Can you work these out from the drawing? Everything is in mm from the part's minimum corner. Coordinates: 2 decimals unless noted, no trailing zeros. Order: outer loops, then holes, each group sorted by start corner. A loop starts at its lowest first (then second) coordinate and runs counter-clockwise, first axis right, second up. Notation, with made-up numbers: (42.5, 34) -> (78.5, 34) arc R19 cw to (78.5, 68) -> close; hole circle Ø4 at (-9.75, 19). An arc over 180 degrees is marked (long way). Return JSON: item names as keys, results as strings. Group by question number.
1) If we section it at D-D, the plane x = 6: Please give me the cut outline in (y, z), then the cut area to 3 significant figures.
2) If I drill on probe 1 along Y at (x, z) = (6, 0.7); probe 2 along Y at (x, z) = (4, 1.15); probe 3 along X at (y, z) = (21.25, 1.8), over which ranges is the centre line in solid material (lowest first)? Write a range as from..to.
3) For pin 1 (4.5 mm diameter, centred on x = 4, y = 20, fed in from +Z); pin 2 (4 mm diameter, centred on x = 15, y = 25, fed in from -Z), each with a flat end and sliding along its axis, tell me the tip position at first contact or that it passes through.
4) If we section it at C-C, the plane y = 25.5: Please give me the cut outline in (x, z), then the cut area to 3 significant figures.
5) If we section it at A-A, the plane x = 36: Please give me the cut outline in (y, z), then the cut area to 3 significant figures.
6) Thinking about a two-plate mould opening in Y: for the marked faces 1, 2 and 3, which applies, +Y half, -Y half, draft (parallel to the pull), parting line (faces both ways), or undercut?
7) If we section it at B-B, the plane z = 1.1: Please give me the cut outline in (x, y).
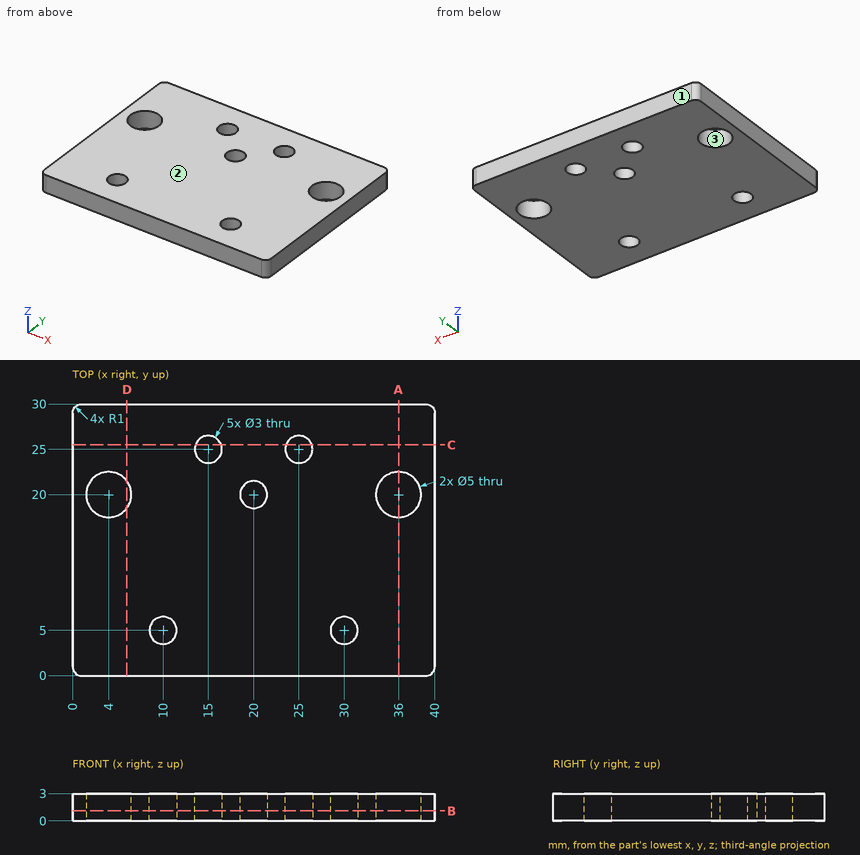
Result sheet:
{
 "1": {"outline": "(0, 0) -> (18.5, 0) -> (18.5, 3) -> (0, 3) -> close; (21.5, 0) -> (30, 0) -> (30, 3) -> (21.5, 3) -> close", "area": "81.0 mm2"},
 "2": {"probe 1": "y = 0..18.5, 21.5..30", "probe 2": "y = 0..17.5, 22.5..30", "probe 3": "x = 0..1.83, 6.17..19.17, 20.83..33.83, 38.17..40"},
 "3": {"pin 1": "passes through", "pin 2": "stops at z = 0"},
 "4": {"outline": "(0, 0) -> (13.59, 0) -> (13.59, 3) -> (0, 3) -> close; (16.41, 0) -> (23.59, 0) -> (23.59, 3) -> (16.41, 3) -> close; (26.41, 0) -> (40, 0) -> (40, 3) -> (26.41, 3) -> close", "area": "103 mm2"},
 "5": {"outline": "(0, 0) -> (17.5, 0) -> (17.5, 3) -> (0, 3) -> close; (22.5, 0) -> (30, 0) -> (30, 3) -> (22.5, 3) -> close", "area": "75.0 mm2"},
 "6": {"face 1": "+Y half", "face 2": "draft", "face 3": "undercut"},
 "7": {"outline": "(0, 1) arc R1 ccw to (1, 0) -> (39, 0) arc R1 ccw to (40, 1) -> (40, 29) arc R1 ccw to (39, 30) -> (1, 30) arc R1 ccw to (0, 29) -> close; hole circle Ø5 at (4, 20); hole circle Ø3 at (10, 5); hole circle Ø3 at (15, 25); hole circle Ø3 at (20, 20); hole circle Ø3 at (25, 25); hole circle Ø3 at (30, 5); hole circle Ø5 at (36, 20)"}
}
